Here's how the part is built. I have some questions about the finished solid (model axes, mm). A direction names the side the tool comes from. Give positions to 0.01 mm unless a question says otherwise; leave off trailing zeros. Loops run counter-clockwise (first coordinate to the right, second up) from the corner with the lowest first, then second, coordinate; pieces in that order, holes last.
Q1. If we section it at C-C (x = 28.5): Please give me the cut outline in (y, z), plus the area to 3 significant figures.
Q2. If we section it at B-B (z = 19.5): Please give me the cut outline in (x, y).
Q3. Will these pins go through, and if not, where does the flat tip stop? P1, Ø1.5, axis at y = 0.5, z = -10.5, coming from the -X side; P2, Ø3.5, axis at x = -7.17, z = 9.17, coming from the +Y side; P3, Ø1.5, axis at x = 22, y = 2.5, coming from the -Z side; P4, Ø2.5, axis at y = 1.5, z = -18.5, coming from the -X side.
Q4. We'd pull the mould along X, two halves only. Please class faces 1 (the face through (3, 2, 59.175)), 2 (the face through (-7.173, 2, -18)), 3 (the face through (-34.673, 4, 19)), 4 (the face through (36.327, 4, 19)): +X half, -X half, draft (parallel to the pull), parting line (faces both ways), or undercut.
Q5. If we section it at A-A (y = 1.4): Please give me the cut outline in (x, z), plus the area to 3 significant figures.
Q6. I need wall thicknesses on line 1 (X direction, y = 3.9, z = 16.5); line 2 (Z direction, x = 12, y = 2.1); line 3 (X direction, y = 4.2, z = 24). Which ranges of each line are inside material? Lowest first, please.
Q7. For faces 5 (the face through (3, 4, -18.325)), 6 (the face through (-6.57, 2.46, 31.08)), 7 (the face through (12.827, 2, 57)), 8 (the face through (12.827, 2, -18)), 9 (the face through (-35, 2, 29.175)), which set-ups out of +Z, -Z, +X, -X, +Y, -Y let a thin tool reach every point of the face, with its end or its side?
Q8. If we section it at D-D (z = -6): Please give me the cut outline in (x, y).
from build123d import *

# Parameters (mm, degrees)
SKETCH1_R           = 2
BOSS_EXTRUDE1_DEPTH = 5
SKETCH2_W           = 4.72967701
SKETCH2_H           = 13.394822952
SKETCH2_W_2         = 13.394822952
SKETCH2_H_2         = 4.72967701
SKETCH2_W_3         = 4.729677011
BOSS_EXTRUDE2_DEPTH = 2.5


with BuildPart() as part:
    # Sketch1 → Boss-Extrude1 (new body)
    with BuildSketch(Plane(origin=(0, 0, 0), x_dir=(1, 0, 0), z_dir=(0, 1, 0))):
        with BuildLine():
            Line((-7.172850367, 15.825076528), (-7.172850367, 20.825076528))
            Line((-7.172850367, 20.825076528), (12.827149633, 20.825076528))
            Line((12.827149633, 20.825076528), (12.827149633, 15.825076528))
            ThreePointArc((12.827149633, 15.825076528), (20.149480103, -1.852593001), (37.827149633, -9.174923472))
            Line((37.827149633, -9.174923472), (42.827149633, -9.174923472))
            Line((42.827149633, -9.174923472), (42.827149633, -29.174923472))
            Line((42.827149633, -29.174923472), (37.827149633, -29.174923472))
            ThreePointArc((37.827149633, -29.174923472), (20.149480103, -36.497253942), (12.827149633, -54.174923472))
            Line((12.827149633, -54.174923472), (12.827149633, -59.174923472))
            Line((12.827149633, -59.174923472), (-7.172850367, -59.174923472))
            Line((-7.172850367, -59.174923472), (-7.172850367, -54.174923472))
            ThreePointArc((-7.172850367, -54.174923472), (-14.495180838, -36.497253942), (-32.172850367, -29.174923472))
            Line((-32.172850367, -29.174923472), (-37.172850367, -29.174923472))
            Line((-37.172850367, -29.174923472), (-37.172850367, -9.174923472))
            Line((-37.172850367, -9.174923472), (-32.172850367, -9.174923472))
            ThreePointArc((-32.172850367, -9.174923472), (-14.495180838, -1.852593001), (-7.172850367, 15.825076528))
        make_face()
        with Locations(Location((-7.172850367, -9.174923472, 0), (0, 0, 270))):
            Circle(SKETCH1_R, mode=Mode.SUBTRACT)
        with Locations(Location((12.827149633, -9.174923472, 0), (0, 0, 270))):
            Circle(SKETCH1_R, mode=Mode.SUBTRACT)
        with Locations(Location((12.827149633, -29.174923472, 0), (0, 0, 270))):
            Circle(SKETCH1_R, mode=Mode.SUBTRACT)
        with Locations(Location((-7.172850367, -29.174923472, 0), (0, 0, 270))):
            Circle(SKETCH1_R, mode=Mode.SUBTRACT)
        with BuildLine():
            Line((-0.922850367, 18.325076528), (6.577149633, 18.325076528))
            ThreePointArc((6.577149633, 18.325076528), (8.577149633, 16.325076528), (6.577149633, 14.325076528))
            Line((6.577149633, 14.325076528), (-0.922850367, 14.325076528))
            ThreePointArc((-0.922850367, 14.325076528), (-2.922850367, 16.325076528), (-0.922850367, 18.325076528))
        make_face(mode=Mode.SUBTRACT)
        with BuildLine():
            Line((36.327149633, -15.424923472), (36.327149633, -22.924923472))
            ThreePointArc((36.327149633, -22.924923472), (38.327149633, -24.924923472), (40.327149633, -22.924923472))
            Line((40.327149633, -22.924923472), (40.327149633, -15.424923472))
            ThreePointArc((40.327149633, -15.424923472), (38.327149633, -13.424923472), (36.327149633, -15.424923472))
        make_face(mode=Mode.SUBTRACT)
        with BuildLine():
            Line((6.577149633, -52.674923472), (-0.922850367, -52.674923472))
            ThreePointArc((-0.922850367, -52.674923472), (-2.922850367, -54.674923472), (-0.922850367, -56.674923472))
            Line((-0.922850367, -56.674923472), (6.577149633, -56.674923472))
            ThreePointArc((6.577149633, -56.674923472), (8.577149633, -54.674923472), (6.577149633, -52.674923472))
        make_face(mode=Mode.SUBTRACT)
        with BuildLine():
            Line((-30.672850367, -22.924923472), (-30.672850367, -15.424923472))
            ThreePointArc((-30.672850367, -15.424923472), (-32.672850367, -13.424923472), (-34.672850367, -15.424923472))
            Line((-34.672850367, -15.424923472), (-34.672850367, -22.924923472))
            ThreePointArc((-34.672850367, -22.924923472), (-32.672850367, -24.924923472), (-30.672850367, -22.924923472))
        make_face(mode=Mode.SUBTRACT)
    extrude(amount=BOSS_EXTRUDE1_DEPTH)

    # Sketch2 → Boss-Extrude2 (add)
    with BuildSketch(Plane.XZ):
        with Locations((38.392291652, 19.174923472)):
            Rectangle(SKETCH2_W, SKETCH2_H)
        with Locations((2.827149633, 54.740065491)):
            Rectangle(SKETCH2_W_2, SKETCH2_H_2)
        with Locations((2.827149633, -16.390218547)):
            Rectangle(SKETCH2_W_2, SKETCH2_H_2)
        with Locations((-32.737992386, 19.174923472)):
            Rectangle(SKETCH2_W_3, SKETCH2_H)
    extrude(amount=-BOSS_EXTRUDE2_DEPTH)


solid = part.part
Check sheet entries:
1. outline: (0, 7.37) - (5, 7.37) - (5, 30.98) - (0, 30.98) - close
1. area: 118 mm2
2. outline: (-37.17, 0) - (42.83, 0) - (42.83, 5) - (40.33, 5) - (40.33, 2.5) - (36.33, 2.5) - (36.33, 5) - (-30.67, 5) - (-30.67, 2.5) - (-34.67, 2.5) - (-34.67, 5) - (-37.17, 5) - close
3. P1: stops at x = -7.92
3. P2: passes through
3. P3: stops at z = 2.89
3. P4: stops at x = -7.17
4. face 1: draft
4. face 2: -X half
4. face 3: undercut
4. face 4: undercut
5. outline: (-37.17, 9.17) - (-32.17, 9.17) arc R25 cw to (-7.17, -15.83) - (-7.17, -20.83) - (12.83, -20.83) - (12.83, -15.83) arc R25 cw to (37.83, 9.17) - (42.83, 9.17) - (42.83, 29.17) - (37.83, 29.17) arc R25 cw to (12.83, 54.17) - (12.83, 59.17) - (-7.17, 59.17) - (-7.17, 54.17) arc R25 cw to (-32.17, 29.17) - (-37.17, 29.17) - close; hole circle Ø4 at (-7.17, 9.17); hole circle Ø4 at (-7.17, 29.17); hole circle Ø4 at (12.83, 9.17); hole circle Ø4 at (12.83, 29.17)
5. area: 3,290 mm2
6. line 1: x = -37.17 to -34.67, -30.67 to 36.33, 40.33 to 42.83
6. line 2: z = -20.83 to 7.35, 11 to 27.35, 31 to 59.17
6. line 3: x = -37.17 to -34.36, -30.99 to 36.64, 40.01 to 42.83
7. face 5: +Y
7. face 6: +Y, -Y
7. face 7: +Z, +X, +Y, -Y
7. face 8: -Z, +X, +Y, -Y
7. face 9: +Z, -X, +Y, -Y
8. outline: (-9.18, 0) - (14.84, 0) - (14.84, 5) - (-9.18, 5) - close
